from build123d import *

# Parameters (mm, degrees)
SKETCH006_R   = 6
SKETCH006_R_2 = 2.2
SKETCH006_W   = 2.75
SKETCH006_H   = 2.75
PAD_DEPTH     = 420


with BuildPart() as part:
    # Sketch006 → Pad (new body)
    with BuildSketch(Plane.XY):
        with BuildLine():
            Line((13.982753, 15), (4.1, 15))
            Line((4.1, 15), (4.1, 13))
            Line((4.1, 13), (8.75, 13))
            Line((8.75, 13), (8.75, 11))
            Line((8.75, 11), (6, 8.25))
            Line((6, 8.25), (-6, 8.25))
            Line((-6, 8.25), (-8.75, 11))
            Line((-8.75, 11), (-8.75, 13))
            Line((-8.75, 13), (-4.1, 13))
            Line((-4.1, 13), (-4.1, 15))
            Line((-4.1, 15), (-14, 15))
            ThreePointArc((-14, 15), (-14.707107, 14.707107), (-15, 14))
            Line((-15, 14), (-15, 4.1))
            Line((-15, 4.1), (-13, 4.1))
            Line((-13, 4.1), (-13, 8.75))
            Line((-13, 8.75), (-11, 8.75))
            Line((-11, 8.75), (-8.25, 6))
            Line((-8.25, 6), (-8.25, -6))
            Line((-8.25, -6), (-11, -8.75))
            Line((-11, -8.75), (-13, -8.75))
            Line((-13, -8.75), (-13, -4.1))
            Line((-13, -4.1), (-15, -4.1))
            Line((-15, -4.1), (-15, -13.982753))
            ThreePointArc((-15, -13.982753), (-14.694808, -14.701948), (-13.965517, -14.982159))
            ThreePointArc((-13.965517, -14.982159), (6.213203, -6.213203), (14.982159, 13.965517))
            ThreePointArc((14.982159, 13.965517), (14.701948, 14.694808), (13.982753, 15))
        make_face()
        Circle(SKETCH006_R, mode=Mode.SUBTRACT)
        with Locations((-5.2, -8.5)):
            Circle(SKETCH006_R_2, mode=Mode.SUBTRACT)
        with Locations((8.5, 5.2)):
            Circle(SKETCH006_R_2, mode=Mode.SUBTRACT)
        with Locations((-11.625, 11.625)):
            Rectangle(SKETCH006_W, SKETCH006_H, mode=Mode.SUBTRACT)
    extrude(amount=PAD_DEPTH)


solid = part.part
Design review of the part built by this model. Coordinates are the model's own, in mm. A direction names the side the tool comes from. Round coordinates to 2 decimals unless told otherwise and drop trailing zeros.
1) Draft analysis for pull direction Y (two halves, no side actions). For faces 3 (the flat face through (-4, 7, 0)), 4 (the cylindrical face through (-6, 0, 207)), 5 (the cylindrical face through (5.989, -6.435, 207.06)), state which applies: released by +Y, released by -Y, zero draft, split by the parting line, or undercut.
The answers:
face 3: zero draft
face 4: undercut
face 5: released by -Y
2) Consider section A-A (z = 83.5). Count the separate pieces of the cut face and the enclosed holes in it, plus the area to 3 significant figures.
The answers:
separate pieces: 1
enclosed holes: 4
area: 371 mm2
3) Machinability: for faces 1 (the flat face through (0, 8.25, 207)), 2 (the flat face through (-15, 9, 207)), which of the approach directions +Z, -Z, +X, -X, +Y, -Y give a long, thin tool a straight path to every point of the face, cutting with its end or side? Answer none if there is none.
The answers:
face 1: +Z, -Z
face 2: +Z, -Z, -X, +Y, -Y
4) Clearance check with flat-ended pins moving along their axes: pin 1 Ø3 at (x, y) = (-8, -6) entering from -Z; pin 2 Ø1.6 at (x, z) = (-11.5, 277.5) entering from -Y; pin 3 Ø3.5 at (x, z) = (5.5, 247.5) entering from -Y; pin 4 Ø5 at (x, z) = (-7, 146) entering from -Y. State where each tip first meets the part, or that it passes through.
The answers:
pin 1: stops at z = 0
pin 2: stops at y = -14.88
pin 3: stops at y = -8.42
pin 4: stops at y = -14.49
5) For L1, parallel to X at y = 6.75, z = 29.5; L2, parallel to Y at x = 0, z = 212; L3, parallel to Y at x = 8.5, z = 237, list the stretches that pass through material, from the lowest coordinate up.
The answers:
L1: x = -15 to -13, -9 to 6.94, 10.06 to 13.84
L2: y = -10.98 to -6, 6 to 8.25
L3: y = -3.65 to 3, 7.4 to 10.75, 13 to 15
